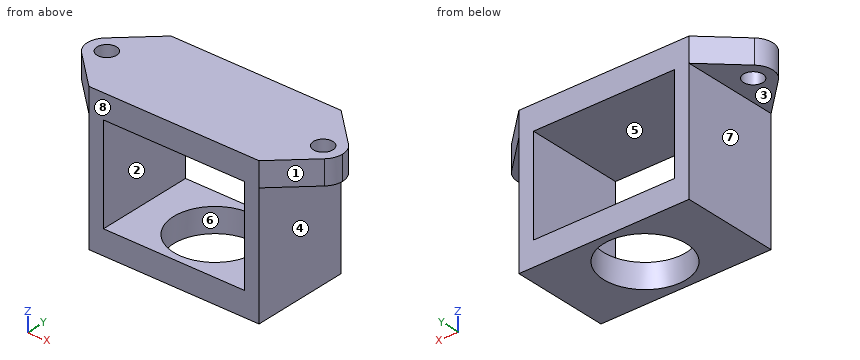
from build123d import *

# Parameters (mm, degrees)
F0_R     = 2
F0_W     = 3
F0_H     = 20
F0_W_2   = 29
F1_DEPTH = 5
F2_DEPTH = 20
F3_W     = 3
F3_H     = 20
F3_W_2   = 32
F3_R     = 8.5
F4_DEPTH = 5


with BuildPart() as f1:
    # F0 (on Top) → F1 (new body)
    with BuildSketch(Plane.XY):
        with BuildLine():
            Line((-17.5, -10), (-17.5, 10))
            Line((-17.5, 10), (-24.9989359016, 2.9057445533))
            ThreePointArc((-24.9989359016, 2.9057445533), (-20.6681883182, 3.6739449919), (-18.25, 0))
            ThreePointArc((-18.25, 0), (-20.6681883182, -3.6739449919), (-24.9989359016, -2.9057445533))
            Line((-24.9989359016, -2.9057445533), (-17.5, -10))
        make_face()
        with BuildLine():
            ThreePointArc((-18.25, 0), (-20.6681883182, 3.6739449919), (-24.9989359016, 2.9057445533))
            ThreePointArc((-24.9989359016, 2.9057445533), (-26.25, 0), (-24.9989359016, -2.9057445533))
            ThreePointArc((-24.9989359016, -2.9057445533), (-20.6681883182, -3.6739449919), (-18.25, 0))
        make_face()
        with Locations((-22.25, 0)):
            Circle(F0_R, mode=Mode.SUBTRACT)
        with Locations((-16, 0)):
            Rectangle(F0_W, F0_H)
        Rectangle(F0_W_2, F0_H)
        with Locations((16, 0)):
            Rectangle(F0_W, F0_H)
        with BuildLine():
            Line((24.9989359016, 2.9057445533), (17.5, 10))
            Line((17.5, 10), (17.5, -10))
            Line((17.5, -10), (24.9989359016, -2.9057445533))
            ThreePointArc((24.9989359016, -2.9057445533), (18.25, 0), (24.9989359016, 2.9057445533))
        make_face()
        with BuildLine():
            ThreePointArc((26.25, 0), (25.9239449919, 1.5818116818), (24.9989359016, 2.9057445533))
            ThreePointArc((24.9989359016, 2.9057445533), (18.25, 0), (24.9989359016, -2.9057445533))
            ThreePointArc((24.9989359016, -2.9057445533), (25.9239449919, -1.5818116818), (26.25, 0))
        make_face()
        with Locations((22.25, 0)):
            Circle(F0_R, mode=Mode.SUBTRACT)
    extrude(amount=F1_DEPTH)

    # F0 (on Top) → F2 (join)
    with BuildSketch(Plane.XY):
        with Locations((-16, 0)):
            Rectangle(F0_W, F0_H)
        with Locations((16, 0)):
            Rectangle(F0_W, F0_H)
    extrude(amount=-F2_DEPTH)

    # F3 (on face) → F4 (join)
    with BuildSketch(Plane(origin=(0, 0, -20), x_dir=(1, 0, 0), z_dir=(0, 0, -1))):
        with Locations((-16, 0)):
            Rectangle(F3_W, F3_H)
        with Locations((1.5, 0)):
            Rectangle(F3_W_2, F3_H)
        Circle(F3_R, mode=Mode.SUBTRACT)
    extrude(amount=F4_DEPTH)


solid = f1.part
The model under review builds one solid part; all positions refer to its coordinate system, in mm. Face numbers are marked on the shaded views. A direction names the side the tool comes from. Round coordinates to 2 decimals unless told otherwise and drop trailing zeros. Loops run counter-clockwise (first coordinate to the right, second up) from the corner with the lowest first, then second, coordinate; pieces in that order, holes last. Notation, with made-up numbers: (-10, -10.75) -> (-2, -10.75) arc R36 ccw to (-2, 25.25) -> close; hole circle Ø11 at (34.25, 20.25). An arc over 180 degrees is marked (long way). Return JSON: item names as keys, results as strings.
(1) For pin 1 (10 mm diameter, centred on y = -2, z = -18.5, fed in from -X); pin 2 (2.5 mm diameter, centred on x = 20.5, y = -3.5, fed in from -Z); pin 3 (6 mm diameter, centred on x = -9, z = -5.5, fed in from +Y); pin 4 (10 mm diameter, centred on y = 2.5, z = -5.5, fed in from +X), all flat-tipped, find the tip position at first contact; note any pin that passes through.
Solved:
{"pin 1": "x = -17.5", "pin 2": "z = 0", "pin 3": "through", "pin 4": "x = 17.5"}
(2) Add section D-D on y = 7.75. Write out the cut boundary in (x, z).
Solved:
{"outline": "(-19.88, 0) -> (-17.5, 0) -> (-17.5, -25) -> (-3.49, -25) -> (-3.49, -20) -> (-14.5, -20) -> (-14.5, 0) -> (14.5, 0) -> (14.5, -20) -> (3.49, -20) -> (3.49, -25) -> (17.5, -25) -> (17.5, 0) -> (19.88, 0) -> (19.88, 5) -> (-19.88, 5) -> close"}
(3) Add section C-C on x = -22.25. Write out the cut boundary in (y, z).
Solved:
{"outline": "(-5.51, 0) -> (-2, 0) -> (-2, 5) -> (-5.51, 5) -> close; (2, 0) -> (5.51, 0) -> (5.51, 5) -> (2, 5) -> close"}
(4) Add section A-A on z = -8.75. Write out the cut boundary in (x, y).
Solved:
{"outline": "(-17.5, -10) -> (-14.5, -10) -> (-14.5, 10) -> (-17.5, 10) -> close; (14.5, -10) -> (17.5, -10) -> (17.5, 10) -> (14.5, 10) -> close"}
(5) For line 1 (Z direction, x = 10.5, y = -9); line 2 (X direction, y = -1, z = -17.5); line 3 (X direction, y = 0, z = -22.35), list the stretches that pass through material, from the lowest coordinate up.
Solved:
{"line 1": "-25 to -20, 0 to 5", "line 2": "-17.5 to -14.5, 14.5 to 17.5", "line 3": "-17.5 to -8.5, 8.5 to 17.5"}
(6) Add section B-B on x = -3.5. Write out the cut boundary in (y, z).
Solved:
{"outline": "(-10, -25) -> (-7.75, -25) -> (-7.75, -20) -> (-10, -20) -> close; (-10, 0) -> (10, 0) -> (10, 5) -> (-10, 5) -> close; (7.75, -25) -> (10, -25) -> (10, -20) -> (7.75, -20) -> close"}
(7) For the marked faces 4, 5, 6, 7 and 8, list the 3-axis set-ups (+Z, -Z, +X, -X, +Y, -Y) from which the entire face can be reached by the end or side of a thin tool; tool diameter is ignored.
Solved:
{"face 4": "-Z, +X, +Y, -Y", "face 5": "+Y, -Y", "face 6": "-Z", "face 7": "-Z, -X, +Y, -Y", "face 8": "+Z, -Z, +X, -X, -Y"}
(8) The part is to be moulded in two halves that separate along Z. For the marked faces 1, 2 and 3, say which applies: released by +Z, released by -Z, zero draft, split by the parting line, or undercut.
Solved:
{"face 1": "zero draft", "face 2": "undercut", "face 3": "released by -Z"}
